Could you check a few things on this model? Use its own coordinates, in mm. Give positions to 0.01 mm unless a question says otherwise; leave off trailing zeros. Order: outer loops, then holes, each group sorted by start corner. A loop starts at its lowest first (then second) coordinate and runs counter-clockwise, first axis right, second up. Notation, with made-up numbers: M -34.75,14.5 L 16.25,14.5 A21 cw 16.25,23.5 Z; hole C 10.25,-12 d8. An arc over 180 degrees is marked long. Use a Markdown table: item, result. Add a question column.
```python
from build123d import *

# Parameters (mm, degrees)
SKETCH1_W               = 230
SKETCH1_H               = 180
BOSS_EXTRUDE1_DEPTH     = 20
FILLET1_R               = 5
SKETCH2_R               = 9
CUT_EXTRUDE1_DEPTH      = 10
SKETCH2_3_R             = 5.5
CUT_EXTRUDE2_DEPTH      = 148.39402973
MIRROR2_COPY_1_SKETCH_R = 9
MIRROR2_COPY_1_DEPTH    = 10
MIRROR2_COPY_2_SKETCH_R = 5.5
MIRROR2_COPY_2_DEPTH    = 148.39402973
FILLET2_R               = 5


with BuildPart() as part:
    # Sketch1 → Boss-Extrude1 (new body)
    with BuildSketch(Plane(origin=(0, 0, 0), x_dir=(1, 0, 0), z_dir=(0, 1, 0))):
        Rectangle(SKETCH1_W, SKETCH1_H)
    extrude(amount=BOSS_EXTRUDE1_DEPTH)

    # Fillet1
    fillet1_edges = [part.edges().sort_by_distance(p)[0] for p in [
        (-115, 20, 0),
        (0, 20, 90),
        (115, 20, 0),
        (0, 20, -90),
    ]]
    fillet(fillet1_edges, radius=FILLET1_R)

    # Sketch2 → Cut-Extrude1 (cut)
    with BuildSketch(Plane.XZ):
        with Locations(Location((-75, 30, 0), (0, 0, 270))):
            Circle(SKETCH2_R)
    cut_extrude1 = extrude(amount=-CUT_EXTRUDE1_DEPTH, mode=Mode.SUBTRACT)

    # Sketch2<3> → Cut-Extrude2 (cut, through all)
    with BuildSketch(Plane.XZ):
        with Locations(Location((-75, 30, 0), (0, 0, 270))):
            Circle(SKETCH2_3_R)
    cut_extrude2 = extrude(amount=-CUT_EXTRUDE2_DEPTH, mode=Mode.SUBTRACT)

    # Mirror1: Cut-Extrude1, Cut-Extrude2 across plane
    add(cut_extrude1.mirror(Plane(origin=(0, 0, 0), x_dir=(0, 0, 1), z_dir=(1, 0, 0))), mode=Mode.SUBTRACT)
    add(cut_extrude2.mirror(Plane(origin=(0, 0, 0), x_dir=(0, 0, 1), z_dir=(1, 0, 0))), mode=Mode.SUBTRACT)

    # Mirror2: Cut-Extrude1, Cut-Extrude2 across plane
    add(cut_extrude1.mirror(Plane.XY), mode=Mode.SUBTRACT)
    add(cut_extrude2.mirror(Plane.XY), mode=Mode.SUBTRACT)

    # Mirror2 copy 1 sketch → Mirror2 copy 1 (cut)
    with BuildSketch(Plane(origin=(0, 0, 0), x_dir=(-1, 0, 0), z_dir=(0, -1, 0))):
        with Locations(Location((-75, 30, 0), (0, 0, 270))):
            Circle(MIRROR2_COPY_1_SKETCH_R)
    extrude(amount=-MIRROR2_COPY_1_DEPTH, mode=Mode.SUBTRACT)

    # Mirror2 copy 2 sketch → Mirror2 copy 2 (cut, through all)
    with BuildSketch(Plane(origin=(0, 0, 0), x_dir=(-1, 0, 0), z_dir=(0, -1, 0))):
        with Locations(Location((-75, 30, 0), (0, 0, 270))):
            Circle(MIRROR2_COPY_2_SKETCH_R)
    extrude(amount=-MIRROR2_COPY_2_DEPTH, mode=Mode.SUBTRACT)

    # Fillet2
    # the kernel refuses this fillet: 5 mm, written as the material it takes off along each edge
    with BuildSketch(Plane(origin=(-110, 15, -85), x_dir=(-1, 0, 0), z_dir=(0, 0, -1))) as fillet2_piece_1_section:
        Polygon((0, 0), (FILLET2_R, 0), (FILLET2_R, FILLET2_R), (0, FILLET2_R), align=None)
    fillet2_piece_1 = extrude(amount=FILLET2_R, mode=Mode.PRIVATE)
    fillet2_piece_1 = fillet2_piece_1 - Plane(origin=(-110, 15, -85), x_dir=(0.7071067811865475, -0.7071067811865475, 0), z_dir=(0, 0, -1)) * Sphere(FILLET2_R, mode=Mode.PRIVATE)
    add(fillet2_piece_1, mode=Mode.SUBTRACT)
    with BuildSketch(Plane(origin=(110, 15, -85), x_dir=(1, 0, 0), z_dir=(0, 0, -1))) as fillet2_piece_2_section:
        Polygon((0, 0), (FILLET2_R, 0), (FILLET2_R, -FILLET2_R), (0, -FILLET2_R), align=None)
    fillet2_piece_2 = extrude(amount=FILLET2_R, mode=Mode.PRIVATE)
    fillet2_piece_2 = fillet2_piece_2 - Plane(origin=(110, 15, -85), x_dir=(-0.7071067811865475, -0.7071067811865475, 0), z_dir=(0, 0, -1)) * Sphere(FILLET2_R, mode=Mode.PRIVATE)
    add(fillet2_piece_2, mode=Mode.SUBTRACT)
    with BuildSketch(Plane(origin=(-110, 15, 85), x_dir=(0, 0, 1), z_dir=(-1, 0, 0))) as fillet2_piece_3_section:
        Polygon((0, 0), (FILLET2_R, 0), (FILLET2_R, FILLET2_R), (0, FILLET2_R), align=None)
    fillet2_piece_3 = extrude(amount=FILLET2_R, mode=Mode.PRIVATE)
    fillet2_piece_3 = fillet2_piece_3 - Plane(origin=(-110, 15, 85), x_dir=(0, -0.7071067811865475, -0.7071067811865475), z_dir=(-1, 0, 0)) * Sphere(FILLET2_R, mode=Mode.PRIVATE)
    add(fillet2_piece_3, mode=Mode.SUBTRACT)
    with BuildSketch(Plane(origin=(110, 15, 85), x_dir=(0, 0, 1), z_dir=(1, 0, 0))) as fillet2_piece_4_section:
        Polygon((0, 0), (FILLET2_R, 0), (FILLET2_R, -FILLET2_R), (0, -FILLET2_R), align=None)
    fillet2_piece_4 = extrude(amount=FILLET2_R, mode=Mode.PRIVATE)
    fillet2_piece_4 = fillet2_piece_4 - Plane(origin=(110, 15, 85), x_dir=(0, -0.7071067811865475, -0.7071067811865475), z_dir=(1, 0, 0)) * Sphere(FILLET2_R, mode=Mode.PRIVATE)
    add(fillet2_piece_4, mode=Mode.SUBTRACT)
    with BuildSketch(Plane(origin=(115, -12.5, 90), x_dir=(0, 0, -1), z_dir=(0, 1, 0)), Plane(origin=(115, -12.5, -90), x_dir=(-1, 0, 0), z_dir=(0, 1, 0))) as fillet2_piece_5:
        with BuildLine():
            CenterArc((FILLET2_R, FILLET2_R), FILLET2_R, 180, 90)
            Line((0, FILLET2_R), (0, 0))
            Line((0, 0), (FILLET2_R, 0))
        make_face()
    extrude(amount=27.5, mode=Mode.SUBTRACT)
    with BuildSketch(Plane(origin=(-115, -12.5, 90), x_dir=(0, 0, -1), z_dir=(0, 1, 0)), Plane(origin=(-115, -12.5, -90), x_dir=(1, 0, 0), z_dir=(0, 1, 0))) as fillet2_piece_6:
        with BuildLine():
            CenterArc((FILLET2_R, -FILLET2_R), FILLET2_R, 90, 90)
            Line((0, -FILLET2_R), (0, 0))
            Line((0, 0), (FILLET2_R, 0))
        make_face()
    extrude(amount=27.5, mode=Mode.SUBTRACT)


solid = part.part
```
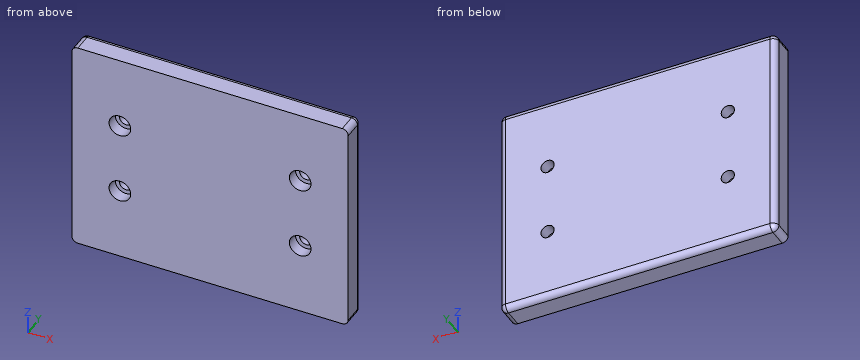
1) Please list where these lines run through material, in increasing order: line 1 (Z direction, x = 75, y = 7.5); line 2 (X direction, y = 4.25, z = -30); line 3 (Z direction, x = 80, y = 16). Write a range as from..to.
2) For pin 1 (16 mm diameter, centred on x = -75, z = -30, fed in from -Y), with a flat end and sliding along its axis, tell me the tip position at first contact or that it passes through.
3) Suppose I cut it at C-C on y = 7.5. Please give me the cut outline in (x, z).
4) Suppose I cut it at B-B on z = -30. Please give me the cut outline in (x, y).
5) Suppose I cut it at A-A on x = 75. Please give me the cut outline in (y, z).
Values found:
| question | item | result |
|---|---|---|
| 1 | line 1 | z = -90..-39, -21..21, 39..90 |
| 1 | line 2 | x = -115..-84, -66..66, 84..115 |
| 1 | line 3 | z = -89.9..-32.29, -27.71..27.71, 32.29..89.9 |
| 2 | pin 1 | stops at y = 10 |
| 3 | outline | M -115,-85 A5 ccw -110,-90 L 110,-90 A5 ccw 115,-85 L 115,85 A5 ccw 110,90 L -110,90 A5 ccw -115,85 Z; hole C -75,-30 d18; hole C -75,30 d18; hole C 75,-30 d18; hole C 75,30 d18 |
| 4 | outline | M -115,0 L -84,0 L -84,10 L -80.5,10 L -80.5,20 L -110,20 A5 ccw -115,15 Z; M -69.5,10 L -66,10 L -66,0 L 66,0 L 66,10 L 69.5,10 L 69.5,20 L -69.5,20 Z; M 80.5,10 L 84,10 L 84,0 L 115,0 L 115,15 A5 ccw 110,20 L 80.5,20 Z |
| 5 | outline | M 0,-90 L 15,-90 A5 ccw 20,-85 L 20,-35.5 L 10,-35.5 L 10,-39 L 0,-39 Z; M 0,-21 L 10,-21 L 10,-24.5 L 20,-24.5 L 20,24.5 L 10,24.5 L 10,21 L 0,21 Z; M 0,39 L 10,39 L 10,35.5 L 20,35.5 L 20,85 A5 ccw 15,90 L 0,90 Z |
